Can you work these out from the model? Positions are in its coordinate system, mm. Face numbers are marked on the shaded views. A direction names the side the tool comes from. Round coordinates to 2 decimals unless told otherwise and drop trailing zeros. Write each loop counter-clockwise with the first axis right and the second up, starting at its lowest first coordinate (ties: lowest second). Pieces come first, ordered by that corner, then holes. Notation, with made-up numbers: (88.25, -30.75) - (102.25, -30.75) arc R10 ccw to (102.25, -22.75) - close; hole circle Ø7 at (62, -31). An arc over 180 degrees is marked (long way). One line per item, written item: value. Start each with the question number.
(1) If I drill on L1, parallel to Y at x = 5, z = 25; L2, parallel to Z at x = 8, y = 25; L3, parallel to X at y = -23.5, z = 5.5, over which ranges is the centre line in solid material (lowest first)? Write a range as from..to.
(2) I want a section at A-A on y = -25. List the corners of the cut face in (x, z) for me, plus the area to 3 significant figures.
(3) I want a section at C-C on z = 0. List the corners of the cut face in (x, y) for me.
(4) I want a section at D-D on y = 0. List the corners of the cut face in (x, z) for me, plus the area to 3 significant figures.
(5) I want a section at B-B on z = -25. List the corners of the cut face in (x, y) for me.
(6) I'm going to push flat-ended pins straight in: pin 1 Ø10 at (x, y) = (22.5, -2) entering from -Z; pin 2 Ø4 at (y, z) = (-25, 25) entering from -X; pin 3 Ø12 at (y, z) = (19, -29.5) entering from +X; pin 4 Ø4 at (y, z) = (-17, -13.5) entering from -X. Where does each tip first touch, or does it pass through?
(7) On a 3-axis mill with a long thin cutter (end or side, diameter ignored), from which of +Z, -Z, +X, -X, +Y, -Y can I reach the whole of each face in a straight line? I mean the marked faces 1, 2 and 3. Say none if no direction works.
from build123d import *

# Parameters (mm, degrees)
SKETCH1_W                = 80
SKETCH1_H                = 70
BOSS_EXTRUDE1_DEPTH      = 10
BOSS_EXTRUDE2_DEPTH      = 50
BOSS_EXTRUDE2_DEPTH_BACK = 25
SKETCH2_R                = 15
LPATTERN1_COUNT          = 2
LPATTERN1_PITCH          = 50
LPATTERN1_COUNT_DIR2     = 2
LPATTERN1_PITCH_DIR2     = 50


with BuildPart() as part:
    # Sketch1 → Boss-Extrude1 (new body)
    with BuildSketch(Plane(origin=(0, 0, 0), x_dir=(0, 0, -1), z_dir=(1, 0, 0))):
        Rectangle(SKETCH1_W, SKETCH1_H)
    extrude(amount=BOSS_EXTRUDE1_DEPTH)

    # Sketch2 → Boss-Extrude2 (add, two sides: drawn at the far end of the back side and taken through both)
    with BuildSketch(Plane(origin=(10, 0, 0), x_dir=(0, 0, -1), z_dir=(1, 0, 0)).offset(-BOSS_EXTRUDE2_DEPTH_BACK)):
        Circle(SKETCH2_R)
    extrude(amount=BOSS_EXTRUDE2_DEPTH + BOSS_EXTRUDE2_DEPTH_BACK)

    # Sketch4 → 1/4 Clearance Hole1 (revolve, cut)
    with BuildSketch(Plane(origin=(10, 25, 25), x_dir=(0, 0, -1), z_dir=(0, 1, 0))):
        Polygon((0, 0), (0, 31.239827343), (3.3782, 29.21), (3.3782, 0), align=None)
    f_1_4_clearance_hole1 = revolve(axis=Axis((16.35, 25, 25), (-1, 0, 0)), mode=Mode.SUBTRACT)

    # LPattern1: 1_4 Clearance Hole1 2 × 2
    with Locations(*[(0, -j * LPATTERN1_PITCH_DIR2, -i * LPATTERN1_PITCH) for i in range(LPATTERN1_COUNT) for j in range(LPATTERN1_COUNT_DIR2) if (i, j) != (0, 0)]):
        add(f_1_4_clearance_hole1, mode=Mode.SUBTRACT)


solid = part.part
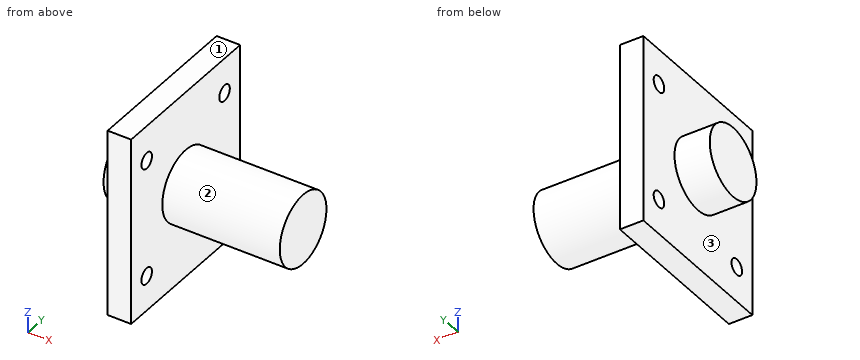
Established:
1. L1: -35..-28.38, -21.62..21.62, 28.38..35
1. L2: -40..-28.38, -21.62..21.62, 28.38..40
1. L3: 0..10
2. outline: (0, -40) - (10, -40) - (10, -28.38) - (0, -28.38) - close; (0, -21.62) - (10, -21.62) - (10, 21.62) - (0, 21.62) - close; (0, 28.38) - (10, 28.38) - (10, 40) - (0, 40) - close
2. area: 665 mm2
3. outline: (-15, -15) - (0, -15) - (0, -35) - (10, -35) - (10, -15) - (60, -15) - (60, 15) - (10, 15) - (10, 35) - (0, 35) - (0, 15) - (-15, 15) - close
4. outline: (-15, -15) - (0, -15) - (0, -40) - (10, -40) - (10, -15) - (60, -15) - (60, 15) - (10, 15) - (10, 40) - (0, 40) - (0, 15) - (-15, 15) - close
4. area: 2,750 mm2
5. outline: (0, -35) - (10, -35) - (10, -28.38) - (0, -28.38) - close; (0, -21.62) - (10, -21.62) - (10, 21.62) - (0, 21.62) - close; (0, 28.38) - (10, 28.38) - (10, 35) - (0, 35) - close
6. pin 1: z = -15
6. pin 2: through
6. pin 3: x = 10
6. pin 4: x = 0
7. face 1: +Z, +X, -X, +Y, -Y
7. face 2: +X
7. face 3: -X
